Check sheet for the modelled part. Datum: model origin and axes. Units: mm. Face numbers are marked on the shaded views. Give positions to 0.01 mm unless a question says otherwise; leave off trailing zeros. Loops run counter-clockwise (first coordinate to the right, second up) from the corner with the lowest first, then second, coordinate; pieces in that order, holes last. Notation, with made-up numbers: (39.25, 5) - (95.25, 5) arc R23 cw to (95.25, 41) - close; hole circle Ø8 at (-34.5, 56.25). An arc over 180 degrees is marked (long way). Use CSV: the item, a comma, the result in double quotes.
from build123d import *

# Parameters (mm, degrees)
BASE_EXTRUDE_DEPTH  = 105
BASE_EXTRUDE_DRAFT  = -1
BOSS_EXTRUDE1_DEPTH = 2.5
CUT_EXTRUDE1_DEPTH  = 105
CUT_EXTRUDE1_DRAFT  = -1


with BuildPart() as part:
    # Sketch1 → Base-Extrude (with draft: the straight prism first)
    with BuildSketch(Plane.XY):
        with BuildLine():
            ThreePointArc((27, 10.394421907), (35.038693587, 15.093935147), (34.887046373, 24.404306911))
            ThreePointArc((34.887046373, 24.404306911), (0, 44.044421907), (-34.887046373, 24.404306911))
            ThreePointArc((-34.887046373, 24.404306911), (-35.038693587, 15.093935147), (-27, 10.394421907))
            Line((-27, 10.394421907), (-13.793114224, 10.394421907))
            ThreePointArc((-13.793114224, 10.394421907), (0, 18.394421907), (13.793114224, 10.394421907))
            Line((13.793114224, 10.394421907), (27, 10.394421907))
        make_face()
    extrude(amount=-BASE_EXTRUDE_DEPTH)
    # Base-Extrude: the draft: its side faces are tilted about the plane it starts from
    base_extrude_sides = [part.faces().sort_by_distance(p)[0] for p in [
        (20.396557112, 10.394421907, -52.5),
        (35.038693587, 15.093935147, -52.5),
        (0, 44.044421907, -52.5),
        (-35.038693587, 15.093935147, -52.5),
        (-20.396557112, 10.394421907, -52.5),
        (0, 18.394421907, -52.5),
    ]]
    draft(base_extrude_sides, Plane.XY, BASE_EXTRUDE_DRAFT)

    # Sketch2 → Boss-Extrude1 (add)
    with BuildSketch(Plane.XY):
        with BuildLine():
            Line((7.889866919, 2.394421907), (27, 2.394421907))
            ThreePointArc((27, 2.394421907), (42.009918378, 11.169393783), (41.726761385, 28.553800683))
            ThreePointArc((41.726761385, 28.553800683), (0, 52.044421907), (-41.726761385, 28.553800683))
            ThreePointArc((-41.726761385, 28.553800683), (-42.009918378, 11.169393783), (-27, 2.394421907))
            Line((-27, 2.394421907), (-7.889866919, 2.394421907))
            ThreePointArc((-7.889866919, 2.394421907), (0, 10.394421907), (7.889866919, 2.394421907))
        make_face()
    extrude(amount=BOSS_EXTRUDE1_DEPTH)


with BuildPart() as cut_extrude1_tool:
    # Sketch4 → Cut-Extrude1 (with draft: the straight prism first)
    with BuildSketch(Plane.XY.offset(2.5)):
        with BuildLine():
            Line((-27, 12.894421907), (-15.173990905, 12.894421907))
            ThreePointArc((-15.173990905, 12.894421907), (0, 20.894421907), (15.173990905, 12.894421907))
            Line((15.173990905, 12.894421907), (27, 12.894421907))
            ThreePointArc((27, 12.894421907), (32.86018584, 16.320354323), (32.749635432, 23.107590108))
            ThreePointArc((32.749635432, 23.107590108), (0, 41.544421907), (-32.749635432, 23.107590108))
            ThreePointArc((-32.749635432, 23.107590108), (-32.86018584, 16.320354323), (-27, 12.894421907))
        make_face()
    extrude(amount=-CUT_EXTRUDE1_DEPTH)
    # Cut-Extrude1: the draft: its side faces are tilted about the plane it starts from
    cut_extrude1_sides = [cut_extrude1_tool.faces().sort_by_distance(p)[0] for p in [
        (-21.086995453, 12.894421907, -50),
        (0, 20.894421907, -50),
        (21.086995453, 12.894421907, -50),
        (32.86018584, 16.320354323, -50),
        (0, 41.544421907, -50),
        (-32.86018584, 16.320354323, -50),
    ]]
    draft(cut_extrude1_sides, Plane.XY.offset(2.5), CUT_EXTRUDE1_DRAFT)


with BuildPart() as part_1:
    add(part.part)

    # Cut-Extrude1: cut by cut_extrude1_tool
    add(cut_extrude1_tool.part, mode=Mode.SUBTRACT)

    # Boss-Extrude2 cone 1 section (through the dimple's axis) → Boss-Extrude2 (revolve)
    with BuildSketch(Plane(origin=(29.717139782, 16.873028946, -105), x_dir=(0, -1, 0), z_dir=(1, 0, 0))):
        Polygon((0, 0), (1.4, 0), (0, 1.4), align=None)
    revolve(axis=Axis((29.717139782, 16.873028946, -105), (0, 0, -1)))


solid = part_1.part
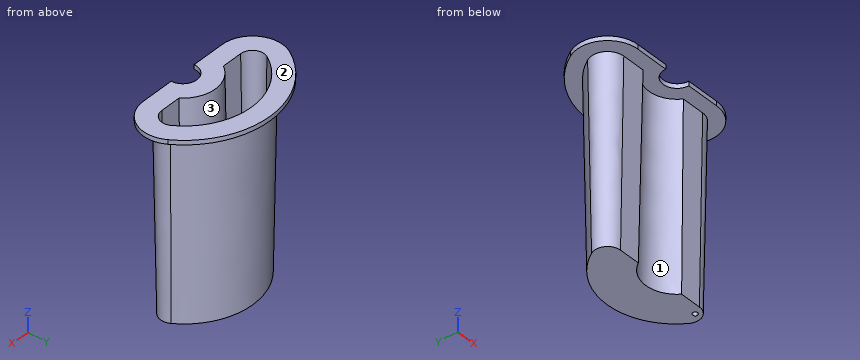
1. Sectioned sample at B-B, the plane z = -37. Record the boundary of the cut face in (x, y).
Completed:
outline,"(-34.33, 24.07) arc R8.58 ccw to (-27, 11.04) - (-14.16, 11.04) arc R16.54 cw to (14.16, 11.04) - (27, 11.04) arc R8.58 ccw to (34.33, 24.07) arc R40.16 ccw to start; hole (-32.16, 22.75) arc R6.04 ccw to (-27, 13.58) - (-15.53, 13.58) arc R19.08 cw to (15.53, 13.58) - (27, 13.58) arc R6.04 ccw to (32.16, 22.75) arc R37.62 ccw to start"
2. Scan lines: line 1 along X through (y, z) = (16, -38.5); line 2 along X through (y, z) = (19.5, -54.5); line 3 along Z through (x, y) = (-17.5, 43). Record each from-to range of solid material in increasing order.
Completed:
line 1,"x = -34.75 to -31.8, -13.52 to -9.6, 9.6 to 13.52, 31.8 to 34.75"
line 2,"x = -35.27 to -32.73, -9.32 to 9.32, 32.73 to 35.27"
line 3,"z = 0 to 2.5"
3. Sectioned sample at C-C, the plane x = -37.5. Record the boundary of the cut face in (y, z).
Completed:
outline,"(5.96, 0) - (34.48, 0) - (34.48, 2.5) - (5.96, 2.5) - close"
4. Sectioned sample at A-A, the plane z = -62. Record the boundary of the cut face in (x, y).
Completed:
outline,"(-33.96, 23.84) arc R8.14 ccw to (-27, 11.48) - (-14.41, 11.48) arc R16.97 cw to (14.41, 11.48) - (27, 11.48) arc R8.14 ccw to (33.96, 23.84) arc R39.72 ccw to start; hole (-31.79, 22.52) arc R5.6 ccw to (-27, 14.02) - (-15.76, 14.02) arc R19.52 cw to (15.76, 14.02) - (27, 14.02) arc R5.6 ccw to (31.79, 22.52) arc R37.18 ccw to start"
5. Release check for a two-part mould opening along X. For the marked faces 1, 2 and 3 record: released by +X, released by -X, zero draft, split by the parting line, or undercut.
Completed:
face 1,"undercut"
face 2,"zero draft"
face 3,"undercut"
6. Go/stop test with flat-tipped pins: pin 1 Ø4 at (x, z) = (-30, -87) entering from -Y; pin 2 Ø1.5 at (x, z) = (-22, -13.5) entering from -Y; pin 3 Ø1 at (y, z) = (19.5, -47) entering from +X. Record where each tip stops, or that it passes through.
Completed:
pin 1,"stops at y = 11.98"
pin 2,"stops at y = 10.62"
pin 3,"stops at x = 35.41"
